Check sheet for the modelled part. Datum: model origin and axes. Units: mm. A direction names the side the tool comes from. Round coordinates to 2 decimals unless told otherwise and drop trailing zeros. Write each loop counter-clockwise with the first axis right and the second up, starting at its lowest first coordinate (ties: lowest second). Pieces come first, ordered by that corner, then holes. Notation, with made-up numbers: (-26.75, 34) -> (23.25, 34) arc R24 ccw to (23.25, 69) -> close; hole circle Ø7 at (50, 31.5). An arc over 180 degrees is marked (long way). One line per item, written item: value.
from build123d import *

# Parameters (mm, degrees)
F0_R     = 15.5
F1_DEPTH = 11.5
F2_R     = 18
F3_DEPTH = 1
F4_R     = 18
F5_DEPTH = 1
F6_R     = 12
F7_DEPTH = 6
F8_R     = 4
F9_DEPTH = 19.501


with BuildPart() as f1:
    # F0 (on Top) → F1 (new body)
    with BuildSketch(Plane.XY):
        Circle(F0_R)
    extrude(amount=F1_DEPTH)

    # F2 (on face) → F3 (join)
    with BuildSketch(Plane.XY.offset(11.5)):
        Circle(F2_R)
    extrude(amount=F3_DEPTH)

    # F4 (on Top) → F5 (join)
    with BuildSketch(Plane.XY):
        Circle(F4_R)
    extrude(amount=-F5_DEPTH)

    # F6 (on face) → F7 (join)
    with BuildSketch(Plane(origin=(0, 0, -1), x_dir=(1, 0, 0), z_dir=(0, 0, -1))):
        Circle(F6_R)
    extrude(amount=F7_DEPTH)

    # F8 (on face) → F9 (cut, through all)
    with BuildSketch(Plane(origin=(0, 0, -7), x_dir=(1, 0, 0), z_dir=(0, 0, -1))):
        Circle(F8_R)
    extrude(amount=-F9_DEPTH, mode=Mode.SUBTRACT)


solid = f1.part
Item 1: Tool access check on faces 5 (the cylindrical face through (-11.99, -0.53, -3.96)), 6 (the cylindrical face through (-2.018, 15.368, 5.67)), 7 (the flat face through (-3, -3, -7)). Record the directions out of +Z, -Z, +X, -X, +Y, -Y that give a thin tool (end or side, any length) a straight path to the whole face; none if there is none.
Answer:
face 5: -Z
face 6: none
face 7: -Z, +X, -X, +Y, -Y
Item 2: Sectioned sample at D-D on x = 14. Enter the section's corners in (y, z).
Answer:
outline: (-11.31, -1) -> (11.31, -1) -> (11.31, 0) -> (6.65, 0) -> (6.65, 11.5) -> (11.31, 11.5) -> (11.31, 12.5) -> (-11.31, 12.5) -> (-11.31, 11.5) -> (-6.65, 11.5) -> (-6.65, 0) -> (-11.31, 0) -> close
Item 3: Mould release check, pull along Z, two halves, no side actions. Record for faces 1 (the cylindrical face through (-2.343, 17.847, 11.993)), 2 (the flat face through (5, 15, 0)), 3 (the flat face through (5, 15, 11.5)), 4 (the flat face through (4, -12, -1)): pulls with the +Z half, pulls with the -Z half, needs draft (parallel to the pull), parting line crosses it, or undercut.
Answer:
face 1: needs draft
face 2: undercut
face 3: undercut
face 4: pulls with the -Z half
Item 4: Thickness scan on line 1 (Y direction, x = 0, z = 4.75); line 2 (Z direction, x = 13, y = 9); line 3 (Y direction, x = 3, z = 9). Record the ranges inside material, lowest first.
Answer:
line 1: y = -15.5 to -4, 4 to 15.5
line 2: z = -1 to 0, 11.5 to 12.5
line 3: y = -15.21 to -2.65, 2.65 to 15.21
Item 5: Depth check by flat-ended pin: P1, Ø3, axis at x = -13.5, z = 0, coming from the +Y side; P2, Ø8, axis at y = 7.5, z = -3.5, coming from the +X side; P3, Ø8, axis at x = 7, z = 0, coming from the +Y side; P4, Ø10, axis at x = -10.5, y = 11, coming from the -Z side. Enter the tip coordinate at first touch or a pass-through.
Answer:
P1: stops at y = 13.42
P2: stops at x = 17.46
P3: stops at y = 17.75
P4: stops at z = -7
Item 6: Sectioned sample at A-A on x = 0. Enter the section's corners in (y, z).
Answer:
outline: (-18, -1) -> (-12, -1) -> (-12, -7) -> (-4, -7) -> (-4, 12.5) -> (-18, 12.5) -> (-18, 11.5) -> (-15.5, 11.5) -> (-15.5, 0) -> (-18, 0) -> close; (4, -7) -> (12, -7) -> (12, -1) -> (18, -1) -> (18, 0) -> (15.5, 0) -> (15.5, 11.5) -> (18, 11.5) -> (18, 12.5) -> (4, 12.5) -> close
Item 7: Sectioned sample at C-C on z = 2.5. Enter the section's corners in (x, y).
Answer:
outline: circle Ø31 at (0, 0); hole circle Ø8 at (0, 0)
